Autodesk Inventor part; units mm, degrees
ref_plane "YZ Plane" through (0, 0, 0) normal (1, 0, 0) x (0, 1, 0)
ref_plane "XZ Plane" through (0, 0, 0) normal (0, 1, 0) x (-1, 0, 0)
ref_plane "XY Plane" through (0, 0, 0) normal (0, 0, 1) x (1, 0, 0)
sketch "Sketch1" plane through (0, 0, 0) normal (0, 0, 1) x (1, 0, 0)
  line L0 (0, 0) -> (26.6, 0)
  line L1 (26.6, 0) -> (26.6, 26.6)
  line L2 (26.6, 26.6) -> (0, 26.6)
  line L3 (0, 26.6) -> (0, 0)
  dimension "d0" = 26.6
  dimension "d1" = 26.6
extrude "Extrusion1" add sketch "Sketch1" along normal blind 3.6
chamfer "Chamfer1" distance 2 angle 45 4 edges at (13.3, 26.6, 0) (0, 13.3, 0) (26.6, 13.3, 0) (13.3, 0, 0)
sketch "Sketch2" plane through (0, 0, 0) normal (0, 0, -1) x (-1, 0, 0)
  line L0 (0, 26.6) -> (0, 0) construction
  line L1 (0, 20.5614) -> (-6, 20.5614) construction
  line L2 (-26.6, 26.6) -> (0, 26.6) construction
  line L3 (-7.1317, 26.6) -> (-7.1317, 21.9) construction
  line L4 (-7.1317, 26.6) -> (-2.4317, 26.6) construction
  line L5 (-6, 21.9) -> (-8.5, 21.9) construction
  line L6 (-8.5, 21.9) -> (-8.5, 14.8) construction
  line L7 (-8.5, 14.8) -> (-6, 14.8) construction
  line L8 (-6, 14.8) -> (-6, 21.9) construction
  line L9 (-13.3, 26.6) -> (-13.3, 0) construction
  line L10 (0, 0) -> (-26.6, 0) construction
  line L11 (-20.6, 21.9) -> (-18.1, 21.9) construction
  line L12 (-18.1, 21.9) -> (-18.1, 14.8) construction
  line L13 (-18.1, 14.8) -> (-20.6, 14.8) construction
  line L14 (-20.6, 14.8) -> (-20.6, 21.9) construction
  line L15 (-13.3, 0) -> (-13.3, 4) construction
  line L16 (-13.3, 4) -> (-10.8, 4) construction
  line L17 (-10.8, 4) -> (-15.8, 4) construction
  line L18 (-15.8, 4) -> (-15.8, 9) construction
  line L19 (-15.8, 9) -> (-10.8, 9) construction
  line L20 (-10.8, 9) -> (-10.8, 4) construction
  line L21 (-15.8, 4) -> (-15.8, 7) construction
  line L22 (-10.8, 4) -> (-10.8, 7) construction
  arc A0 (-10.8, 7) -> (-15.8, 7) centre (-13.3, 6.4375) ccw construction
  line L23 (-20.6, 21.9) -> (-18.1, 21.9)
  line L24 (-18.1, 21.9) -> (-18.1, 14.8)
  line L25 (-18.1, 14.8) -> (-20.6, 14.8)
  line L26 (-20.6, 14.8) -> (-20.6, 21.9)
  line L27 (-8.5, 21.9) -> (-6, 21.9)
  line L28 (-6, 21.9) -> (-6, 14.8)
  line L29 (-6, 14.8) -> (-8.5, 14.8)
  line L30 (-8.5, 14.8) -> (-8.5, 21.9)
  line L31 (-15.8, 4) -> (-10.8, 4)
  line L32 (-10.8, 7) -> (-10.8, 4)
  line L33 (-15.8, 4) -> (-15.8, 7)
  arc A1 (-10.8, 7) -> (-15.8, 7) centre (-13.3, 6.4375) ccw
  dimension "d7" = 6
  dimension "d9" = 4.7
  dimension "d11" = 2.5
  dimension "d12" = 7.1
  dimension "d13" = 4
  dimension "d14" = 2.5
  dimension "d15" = 5
  dimension "d16" = 5
  dimension "d17" = 3
extrude "Extrusion2" cut sketch "Sketch2" against normal blind 3.6
sketch "Sketch3" plane through (0, 0, 3.6) normal (0, 0, 1) x (1, 0, 0)
  line L0 (15.8, 4) -> (10.8, 4) construction
  line L1 (10.8, 4) -> (10.8, 7) construction
  arc A0 (15.8, 7) -> (10.8, 7) centre (13.3, 6.4375) ccw construction
  line L2 (15.8, 7) -> (15.8, 4) construction
  line L3 (6, 14.8) -> (6, 21.9) construction
  line L4 (6, 21.9) -> (8.5, 21.9) construction
  line L5 (8.5, 21.9) -> (8.5, 14.8) construction
  line L6 (8.5, 14.8) -> (6, 14.8) construction
  line L7 (18.1, 14.8) -> (18.1, 21.9) construction
  line L8 (18.1, 21.9) -> (20.6, 21.9) construction
  line L9 (20.6, 21.9) -> (20.6, 14.8) construction
  line L10 (20.6, 14.8) -> (18.1, 14.8) construction
  line L11 (26.6, 0) -> (26.6, 26.6) construction
  line L12 (26.6, 26.6) -> (0, 26.6) construction
  line L13 (0, 26.6) -> (0, 0) construction
  line L14 (0, 0) -> (26.6, 0) construction
  line L15 (13.3, 26.6) -> (13.3, 0) construction
  line L16 (4.8, 2.55) -> (21.8, 2.55) construction
  line L17 (21.8, 2.55) -> (21.8, 24.05) construction
  line L18 (21.8, 24.05) -> (4.8, 24.05) construction
  line L19 (4.8, 24.05) -> (4.8, 2.55) construction
  line L20 (4.8, 2.55) -> (21.8, 24.05) construction
  line L21 (21.8, 2.55) -> (4.8, 24.05) construction
  line L22 (21.8, 2.55) -> (17.4, 2.55) construction
  line L23 (17.4, 2.55) -> (17.4, 8.55) construction
  line L24 (17.4, 8.55) -> (21.8, 8.55) construction
  line L25 (21.8, 8.55) -> (21.8, 2.55) construction
  line L26 (4.8, 2.55) -> (9.2, 2.55) construction
  line L27 (9.2, 2.55) -> (9.2, 8.55) construction
  line L28 (9.2, 8.55) -> (4.8, 8.55) construction
  line L29 (4.8, 8.55) -> (4.8, 2.55) construction
  line L30 (11.8, 37.0426) -> (14.8, 37.0426) construction
  line L31 (14.8, 37.0426) -> (14.8, 11.0574) construction
  line L32 (14.8, 11.0574) -> (11.8, 11.0574) construction
  line L33 (11.8, 11.0574) -> (11.8, 37.0426) construction
  line L34 (11.8, 37.0426) -> (14.8, 11.0574) construction
  line L35 (14.8, 37.0426) -> (11.8, 11.0574) construction
  line L36 (4.8, 24.05) -> (11.8, 24.05)
  line L37 (11.8, 11.0574) -> (11.8, 24.05)
  line L38 (11.8, 11.0574) -> (14.8, 11.0574)
  line L39 (14.8, 11.0574) -> (14.8, 24.05)
  line L40 (14.8, 24.05) -> (21.8, 24.05)
  line L41 (21.8, 24.05) -> (21.8, 8.55)
  line L42 (21.8, 8.55) -> (17.4, 8.55)
  line L43 (17.4, 8.55) -> (17.4, 2.55)
  line L44 (17.4, 2.55) -> (9.2, 2.55)
  line L45 (9.2, 2.55) -> (9.2, 8.55)
  line L46 (9.2, 8.55) -> (4.8, 8.55)
  line L47 (4.8, 8.55) -> (4.8, 24.05)
  point P0 (13.3, 13.3)
  point P1 (13.3, 24.05)
  dimension "d20" = 17
  dimension "d21" = 21.5
  dimension "d22" = 4.4
  dimension "d23" = 6
  dimension "d24" = 4.4
  dimension "d25" = 6
  dimension "d26" = 3
extrude "Extrusion3" add sketch "Sketch3" along normal blind 20
chamfer "Chamfer2" distance 1 angle 45 4 edges at (4.8, 24.05, 13.6) (21.8, 24.05, 13.6) (17.4, 2.55, 13.6) (9.2, 2.55, 13.6)
fillet "Fillet1" radius 0.5 13 edges at (8.8, 24.05, 23.6) (4.8, 15.8, 23.6) (11.8, 17.5537, 23.6) (14.8, 17.5537, 23.6) (17.8, 24.05, 23.6) (21.8, 15.8, 23.6) (19.6, 8.55, 23.6) (17.4, 6.05, 23.6) (9.2, 6.05, 23.6) (7, 8.55, 23.6) (13.3, 2.55, 23.6) (21.3, 23.55, 23.6) (5.3, 23.55, 23.6)
ref_plane "Work Plane1" through (14.8, 16.3, 3.6) normal (0, 1, 0) x (1, 0, 0)
sketch "Sketch4" plane through (14.8, 16.3, 3.6) normal (0, 1, 0) x (1, 0, 0)
  line L0 (-10, 0) -> (-10, -19.5) construction
  line L1 (11.8, 0) -> (-14.8, 0) construction
  line L2 (-8.7929, -20) -> (-3.5, -20) construction
  arc A0 (-3.5, -20) -> (-3, -19.5) centre (-3.5, -19.5) ccw construction
  line L3 (-3, -19.5) -> (-9, -19.5) construction
  ellipse E0 centre (-8.7929, -19.5) end of major axis (-8.7929, -20) minor radius 0.2071 (-9, -19.5) -> (-8.7929, -20) ccw construction
  line L4 (-9.5, -20) -> (-8.7929, -20) construction
  ellipse E1 centre (-8.7929, -19.5) end of major axis (-8.7929, -20) minor radius 0.2071 (-9, -19.5) -> (-8.7929, -20) ccw construction
  line L5 (-9, -19.5) -> (-10, -19.5) construction
  arc A1 (-10, -19.5) -> (-9.5, -20) centre (-9.5, -19.5) ccw construction
  line L6 (-7.8516, -20) -> (-7.8516, -17.5) construction
  line L7 (-7.8516, -17.5) -> (-16.9269, -17.5) construction
  line L8 (-10, -3.8087) -> (-15, -3.8087) construction
  line L9 (-14.8, 0) -> (-14.8, -3) construction
  line L10 (-10, 0) -> (-11.6, 0) construction
  line L11 (-11.6, 0) -> (-14.8, -3) construction
  line L12 (-10, -17.5) -> (-12, -17.5) construction
  line L13 (-12, -17.5) -> (-14.8, -3) construction
  arc A2 (-12.3892, -15.4843) -> (-10, -17.5) centre (-10.1078, -15.204) ccw construction
  arc A3 (-12.3892, -15.4843) -> (-10, -17.5) centre (-10.1078, -15.204) ccw
  line L14 (-12.3892, -15.4843) -> (-14.8, -3)
  line L15 (-14.8, -3) -> (-11.6, 0)
  line L16 (-11.6, 0) -> (-10, 0)
  line L17 (-10, 0) -> (-10, -17.5)
  point P0 (-14.8, 3.6)
  dimension "d33" = 2.5
  dimension "d34" = 5
  dimension "d35" = 3
  dimension "d36" = 1.6
  dimension "d37" = 2
extrude "Extrusion4" add sketch "Sketch4" along normal blind 7.3 and the other way blind 3.65
ref_plane "Work Plane2" through (13.3, 11.0574, 3.6) normal (-1, 0, 0) x (0, 0, 1)
mirror "Mirror1" about plane through (13.3, 11.0574, 3.6) normal (-1, 0, 0) of "Extrusion4"
properties part number "Plug"
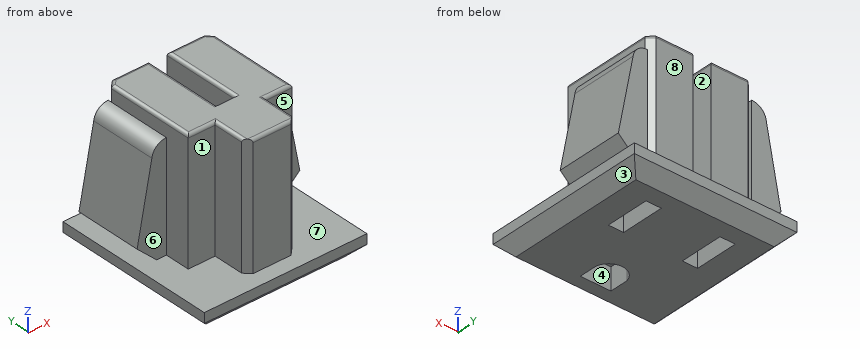
For this review, take the finished solid that the model builds, in its own axes (mm). Face numbers are marked on the shaded views. A direction names the side the tool comes from. Give positions to 0.01 mm unless a question says otherwise; leave off trailing zeros. Order: outer loops, then holes, each group sorted by start corner. A loop starts at its lowest first (then second) coordinate and runs counter-clockwise, first axis right, second up. Notation, with made-up numbers: (-27.75, 45.5) -> (-12.75, 45.5) arc R30 cw to (-12.75, 77.5) -> close; hole circle Ø2 at (73.5, -34.75). An arc over 180 degrees is marked (long way). Write item = value, one per line.
1) Draft analysis for pull direction X (two halves, no side actions). For the marked faces 1, 2 and 3, state which applies: pulls with the +X half, pulls with the -X half, needs draft (parallel to the pull), parting line crosses it, or undercut.
Findings:
face_1 = needs draft
face_2 = undercut
face_3 = pulls with the +X half
2) We need section D-D, the plane y = 6.25. Give the boundary of the cut face in (x, z), and give its area (3 significant figures).
Findings:
outline = (0, 2) -> (2, 0) -> (10.8, 0) -> (10.8, 3.6) -> (15.8, 3.6) -> (15.8, 0) -> (24.6, 0) -> (26.6, 2) -> (26.6, 3.6) -> (17.4, 3.6) -> (17.4, 23.1) arc R0.5 ccw to (16.9, 23.6) -> (9.7, 23.6) arc R0.5 ccw to (9.2, 23.1) -> (9.2, 3.6) -> (0, 3.6) -> close
area = 238 mm^2
3) We need section B-B, the plane x = 7. Give the boundary of the cut face in (y, z), and give its area (3 significant figures).
Findings:
outline = (0, 2) -> (2, 0) -> (14.8, 0) -> (14.8, 3.6) -> (21.9, 3.6) -> (21.9, 0) -> (24.6, 0) -> (26.6, 2) -> (26.6, 3.6) -> (24.05, 3.6) -> (24.05, 23.1) arc R0.5 ccw to (23.55, 23.6) -> (9.05, 23.6) arc R0.5 ccw to (8.55, 23.1) -> (8.55, 3.6) -> (0, 3.6) -> close
area = 376 mm^2
4) We need section C-C, the plane z = 13. Give the boundary of the cut face in (x, y).
Findings:
outline = (1.24, 12.65) -> (4.8, 12.65) -> (4.8, 8.55) -> (9.2, 8.55) -> (9.2, 3.55) -> (10.2, 2.55) -> (16.4, 2.55) -> (17.4, 3.55) -> (17.4, 8.55) -> (21.8, 8.55) -> (21.8, 12.65) -> (25.36, 12.65) -> (25.36, 23.6) -> (21.8, 23.6) -> (21.8, 23.05) -> (20.8, 24.05) -> (14.8, 24.05) -> (14.8, 11.06) -> (11.8, 11.06) -> (11.8, 24.05) -> (5.8, 24.05) -> (4.8, 23.05) -> (4.8, 23.6) -> (1.24, 23.6) -> close
5) To check wall thickness, follow L1, parallel to X at y = 5.25, z = 2; L2, parallel to Z at x = 3, y = 8.5; L3, parallel to Y at x = 18.5, z = 20.25. State the ranges of each line that lie inside material, in increasing order. Write a range as from..to.
Findings:
L1 = 0..10.8, 15.8..26.6
L2 = 0..3.6
L3 = 8.55..24.05
6) For the marked faces 4, 5, 6, 7 and 8, list the 3-axis set-ups (+Z, -Z, +X, -X, +Y, -Y) from which the entire face can be reached by the end or side of a thin tool; tool diameter is ignored.
Findings:
face_4 = -Z
face_5 = +Z, +X, -Y
face_6 = +Z, -X, -Y
face_7 = none
face_8 = +Z, +X, -X, +Y
7) Insertion check: pin 1 (4 mm diameter, centred on y = 5.5, z = 10, fed in from -X); pin 2 (6.5 mm diameter, centred on x = 8, z = 12.5, fed in from +Y); pin 3 (12 mm diameter, centred on x = 17.5, y = 15.5, fed in from -Z); pin 4 (5.5 mm diameter, centred on x = 2, z = 10, fed in from +Y). Each pin has a flat end and moves straight along its axis. Give the tip position at first contact, or say it passes through.
Findings:
pin_1 = 9.2
pin_2 = 24.05
pin_3 = 0
pin_4 = 23.6
